from build123d import *

# Parameters (mm, degrees)
SKETCH_1_R          = 25
SKETCH_1_W          = 115
SKETCH_1_H          = 30
EXTRUDE_1_DEPTH     = 10
FILLET_1_R          = 20
SKETCH_2_R          = 18.75
CUT_EXTRUDE_1_DEPTH = 81.195074662
CUT_EXTRUDE_3_DEPTH = 81.195074662
FILLET_3_R          = 3
SKETCH_5_R          = 1.65
CUT_EXTRUDE_4_DEPTH = 81.195074662
SKETCH_6_R          = 1.65
CUT_EXTRUDE_5_DEPTH = 81.195074662
FILLET_5_R          = 5
SKETCH_7_R          = 18.75
SKETCH_7_R_2        = 16.75
EXTRUDE_2_DEPTH     = 2.3
CUT_EXTRUDE_6_DEPTH = 10
FILLET_6_R          = 3
SKETCH_9_R          = 1.65
CUT_EXTRUDE_7_DEPTH = 10


with BuildPart() as part:
    # ｽｹｯﾁ1 → ﾎﾞｽ - 押し出し1 (new body)
    with BuildSketch(Plane.XY):
        with Locations((30, 30)):
            Circle(SKETCH_1_R)
        with Locations((-30, 30)):
            Circle(SKETCH_1_R)
        Rectangle(SKETCH_1_W, SKETCH_1_H)
        with BuildLine():
            ThreePointArc((-50, 15), (-30, 5), (-10, 15))
            Line((-10, 15), (-50, 15))
        make_face()
        with BuildLine():
            Line((-50, 15), (-10, 15))
            ThreePointArc((-10, 15), (-6.282917549, 22.09430585), (-5, 30))
            ThreePointArc((-5, 30), (-12.32233047, 47.67766953), (-30, 55))
            ThreePointArc((-30, 55), (-47.67766953, 47.67766953), (-55, 30))
            ThreePointArc((-55, 30), (-53.717082451, 22.09430585), (-50, 15))
        make_face()
        with BuildLine():
            Line((-10, 15), (10, 15))
            ThreePointArc((10, 15), (7.639320225, 41.180339887), (30, 55))
            Line((30, 55), (-30, 55))
            ThreePointArc((-30, 55), (-12.32233047, 47.67766953), (-5, 30))
            ThreePointArc((-5, 30), (-6.282917549, 22.09430585), (-10, 15))
        make_face()
        with BuildLine():
            ThreePointArc((10, 15), (30, 5), (50, 15))
            Line((50, 15), (10, 15))
        make_face()
        with BuildLine():
            Line((10, 15), (50, 15))
            ThreePointArc((50, 15), (53.717082451, 22.09430585), (55, 30))
            ThreePointArc((55, 30), (47.67766953, 47.67766953), (30, 55))
            ThreePointArc((30, 55), (7.639320225, 41.180339887), (10, 15))
        make_face()
        with BuildLine():
            Line((50, 15), (57.5, 15))
            Line((57.5, 15), (55, 30))
            ThreePointArc((55, 30), (53.717082451, 22.09430585), (50, 15))
        make_face()
        with BuildLine():
            Line((-55, 30), (-57.5, 15))
            Line((-57.5, 15), (-50, 15))
            ThreePointArc((-50, 15), (-53.717082451, 22.09430585), (-55, 30))
        make_face()
    extrude(amount=EXTRUDE_1_DEPTH)

    # ﾌｨﾚｯﾄ1
    fillet_1_edges = [part.edges().sort_by_distance(p)[0] for p in [
        (55, 30, 5),
        (57.5, 15, 5),
        (-57.5, 15, 5),
        (-55, 30, 5),
    ]]
    fillet(fillet_1_edges, radius=FILLET_1_R)

    # ｽｹｯﾁ2 → ｶｯﾄ - 押し出し1 (cut, through all)
    with BuildSketch(Plane.XY.offset(10)):
        with Locations((30, 30)):
            Circle(SKETCH_2_R)
        with Locations(Location((-30, 30, 0), (0, 0, 180))):
            Circle(SKETCH_2_R)
    extrude(amount=-CUT_EXTRUDE_1_DEPTH, mode=Mode.SUBTRACT)

    # ｽｹｯﾁ4 → ｶｯﾄ - 押し出し3 (cut, through all)
    with BuildSketch(Plane(origin=(0, 0, 0), x_dir=(-1, 0, 0), z_dir=(0, 0, -1))):
        with BuildLine():
            Line((-5, -5), (-5, 15))
            Line((-5, 15), (-10, 15))
            ThreePointArc((-10, 15), (-28.103103333, 5.072068216), (-47.5, 12.146428929))
            Line((-47.5, 12.146428929), (-47.5, -5))
            Line((-47.5, -5), (-5, -5))
        make_face()
        with BuildLine():
            Line((10, 15), (5, 15))
            Line((5, 15), (5, -5))
            Line((5, -5), (47.5, -5))
            Line((47.5, -5), (47.5, 12.146428929))
            ThreePointArc((47.5, 12.146428929), (28.103103333, 5.072068216), (10, 15))
        make_face()
    extrude(amount=-CUT_EXTRUDE_3_DEPTH, mode=Mode.SUBTRACT)

    # ﾌｨﾚｯﾄ3
    fillet_3_edges = [part.edges().sort_by_distance(p)[0] for p in [
        (-47.5, 12.146428929, 5),
        (-47.5, -5, 5),
        (-5, -5, 5),
        (-5, 15, 5),
        (-10, 15, 5),
        (47.5, 12.146428929, 5),
        (10, 15, 5),
        (5, 15, 5),
        (5, -5, 5),
        (47.5, -5, 5),
    ]]
    fillet(fillet_3_edges, radius=FILLET_3_R)

    # ｽｹｯﾁ5 → ｶｯﾄ - 押し出し4 (cut, through all)
    with BuildSketch(Plane(origin=(0, 0, 0), x_dir=(-1, 0, 0), z_dir=(0, 0, -1))):
        with Locations((-30, 51.75)):
            Circle(SKETCH_5_R)
        with Locations((-14.620427509, 45.379572491)):
            Circle(SKETCH_5_R)
        with Locations((-8.25, 30)):
            Circle(SKETCH_5_R)
        with Locations((-14.620427509, 14.620427509)):
            Circle(SKETCH_5_R)
        with Locations((-30, 8.25)):
            Circle(SKETCH_5_R)
        with Locations((-45.379572491, 14.620427509)):
            Circle(SKETCH_5_R)
        with Locations((-51.75, 30)):
            Circle(SKETCH_5_R)
        with Locations((-45.379572491, 45.379572491)):
            Circle(SKETCH_5_R)
        with Locations(Location((45.379572491, 45.379572491, 0), (0, 0, 180))):
            Circle(SKETCH_5_R)
        with Locations(Location((51.75, 30, 0), (0, 0, 180))):
            Circle(SKETCH_5_R)
        with Locations(Location((45.379572491, 14.620427509, 0), (0, 0, 180))):
            Circle(SKETCH_5_R)
        with Locations(Location((30, 8.25, 0), (0, 0, 180))):
            Circle(SKETCH_5_R)
        with Locations(Location((14.620427509, 14.620427509, 0), (0, 0, 180))):
            Circle(SKETCH_5_R)
        with Locations(Location((8.25, 30, 0), (0, 0, 180))):
            Circle(SKETCH_5_R)
        with Locations(Location((14.620427509, 45.379572491, 0), (0, 0, 180))):
            Circle(SKETCH_5_R)
        with Locations(Location((30, 51.75, 0), (0, 0, 180))):
            Circle(SKETCH_5_R)
    extrude(amount=-CUT_EXTRUDE_4_DEPTH, mode=Mode.SUBTRACT)

    # ｽｹｯﾁ6 → ｶｯﾄ - 押し出し5 (cut, through all)
    with BuildSketch(Plane(origin=(0, 0, 0), x_dir=(-1, 0, 0), z_dir=(0, 0, -1))):
        with Locations((-52.5, -10)):
            Circle(SKETCH_6_R)
        with Locations(Location((52.5, -10, 0), (0, 0, 180))):
            Circle(SKETCH_6_R)
        with Locations((0, -5)):
            Circle(SKETCH_6_R)
    extrude(amount=-CUT_EXTRUDE_5_DEPTH, mode=Mode.SUBTRACT)

    # ﾌｨﾚｯﾄ5
    fillet_5_edges = [part.edges().sort_by_distance(p)[0] for p in [
        (57.5, -15, 5),
        (-57.5, -15, 5),
    ]]
    fillet(fillet_5_edges, radius=FILLET_5_R)

    # ｽｹｯﾁ7 → ﾎﾞｽ - 押し出し2 (add)
    # profile 1 of 2: a face of its own
    with BuildSketch(Plane.XY.offset(10)):
        with Locations((-30, 30)):
            Circle(SKETCH_7_R)
        with Locations((-30, 30)):
            Circle(SKETCH_7_R_2, mode=Mode.SUBTRACT)
    # profile 2 of 2: a face of its own
    with BuildSketch(Plane.XY.offset(10)):
        with Locations((30, 30)):
            Circle(SKETCH_7_R)
        with Locations((30, 30)):
            Circle(SKETCH_7_R_2, mode=Mode.SUBTRACT)
    extrude(amount=-EXTRUDE_2_DEPTH)

    # ｽｹｯﾁ8 → ｶｯﾄ - 押し出し6 (cut)
    with BuildSketch(Plane(origin=(0, 0, 0), x_dir=(-1, 0, 0), z_dir=(0, 0, -1))):
        with BuildLine():
            Line((-5.459217616, 20), (0, 20))
            Line((0, 20), (0, 50))
            Line((0, 50), (-12.614661349, 50))
            ThreePointArc((-12.614661349, 50), (-5.886088307, 40.989506944), (-3.5, 30))
            ThreePointArc((-3.5, 30), (-3.994416627, 24.904940293), (-5.459217616, 20))
        make_face()
        with BuildLine():
            Line((0, 50), (0, 20))
            Line((0, 20), (5.459217616, 20))
            ThreePointArc((5.459217616, 20), (4.223074151, 36.148178084), (12.614661349, 50))
            Line((12.614661349, 50), (0, 50))
        make_face()
    extrude(amount=-CUT_EXTRUDE_6_DEPTH, mode=Mode.SUBTRACT)

    # ﾌｨﾚｯﾄ6
    fillet_6_edges = [part.edges().sort_by_distance(p)[0] for p in [
        (-5.459217616, 20, 5),
        (5.459217616, 20, 5),
        (12.614661349, 50, 5),
        (-12.614661349, 50, 5),
    ]]
    fillet(fillet_6_edges, radius=FILLET_6_R)

    # ｽｹｯﾁ9 → ｶｯﾄ - 押し出し7 (cut)
    with BuildSketch(Plane.XZ.offset(15)):
        with Locations((-42.5, 5)):
            Circle(SKETCH_9_R)
        with Locations(Location((42.5, 5, 0), (0, 0, 180))):
            Circle(SKETCH_9_R)
    extrude(amount=-CUT_EXTRUDE_7_DEPTH, mode=Mode.SUBTRACT)


solid = part.part
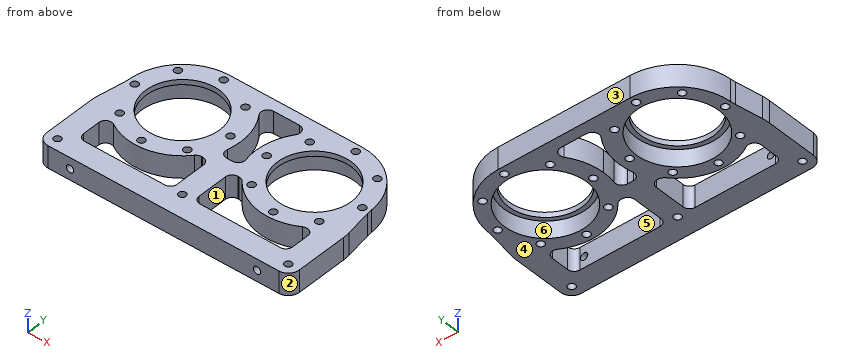
Build history of the part. All positions in model axes, mm. Face numbers are marked on the shaded views. A direction names the side the tool comes from. Round coordinates to 2 decimals unless told otherwise and drop trailing zeros. Loops run counter-clockwise (first coordinate to the right, second up) from the corner with the lowest first, then second, coordinate; pieces in that order, holes last. Notation, with made-up numbers: (56, 4.5) -> (111, 4.5) arc R16 ccw to (111, 10.5) -> close; hole circle Ø11 at (3.25, 35). An arc over 180 degrees is marked (long way). One line per item, written item: value. Start each with the question number.
Q1. Cut at C-C on y = 37.5. List the corners of the cut face in (x, z), plus the area to 3 significant figures.
Q2. Cut at D-D on z = 5. Count the separate pieces of the cut face and the enclosed holes in it, plus the area to 3 significant figures.
Q3. Cut at B-B on y = 1. List the corners of the cut face in (x, z).
Q4. Probe line 1 along X through (y, z) = (2, 4); line 2 along Y through (x, z) = (30, 5.25); line 3 along Y through (x, z) = (-30, 9.5). List the from-to ranges inside material, lowest first.
Q5. Two-plate mould, pull along Y, no slides. Class the marked faces 1, 2 and 3: released by +Y, released by -Y, zero draft, split by the parting line, or undercut.
Q6. Drop flat-ended pins along their axis: pin 1 Ø3 at (x, y) = (-30, 51.75) entering from -Z; pin 2 Ø2 at (x, z) = (42.5, 5) entering from +Y; pin 3 Ø1 at (y, z) = (29.5, 6) entering from +X. Give the stop position or say it passes through.
Q7. Cut at A-A on x = 0. List the corners of the cut face in (y, z), plus the area to 3 significant figures.
Q8. 3-axis set-ups, long thin cutter, end or side, ignore diameter. For the marked faces 4, 5 and 6: which of +Z, -Z, +X, -X, +Y, -Y reach the whole face in a straight line?
Computed:
1. outline: (-53.85, 0) -> (-47.18, 0) -> (-47.18, 7.7) -> (-44.98, 7.7) -> (-44.98, 10) -> (-53.85, 10) -> close; (-15.02, 7.7) -> (-12.82, 7.7) -> (-12.82, 0) -> (-4.58, 0) -> (-4.58, 10) -> (-15.02, 10) -> close; (4.58, 0) -> (12.82, 0) -> (12.82, 7.7) -> (15.02, 7.7) -> (15.02, 10) -> (4.58, 10) -> close; (44.98, 7.7) -> (47.18, 7.7) -> (47.18, 0) -> (53.85, 0) -> (53.85, 10) -> (44.98, 10) -> close
1. area: 318 mm²
2. separate pieces: 1
2. enclosed holes: 22
2. area: 3,740 mm²
3. outline: (-57.5, 0) -> (-47.5, 0) -> (-47.5, 10) -> (-57.5, 10) -> close; (-5, 0) -> (5, 0) -> (5, 10) -> (-5, 10) -> close; (47.5, 0) -> (57.5, 0) -> (57.5, 10) -> (47.5, 10) -> close
4. line 1: -57.5 to -47.5, -5 to 5, 47.5 to 57.5
4. line 2: -15 to -5, 5 to 6.6, 9.9 to 11.25, 48.75 to 50.1, 53.4 to 55
4. line 3: -15 to -5, 5 to 6.6, 9.9 to 13.25, 46.75 to 50.1, 53.4 to 55
5. face 1: undercut
5. face 2: released by -Y
5. face 3: released by +Y
6. pin 1: through
6. pin 2: y = 52.2
6. pin 3: x = 55.17
7. outline: (-15, 0) -> (-6.65, 0) -> (-6.65, 10) -> (-15, 10) -> close; (-3.35, 0) -> (20, 0) -> (20, 10) -> (-3.35, 10) -> close; (50, 0) -> (55, 0) -> (55, 10) -> (50, 10) -> close
7. area: 367 mm²
8. face 4: -Z, +X, -X, +Y, -Y
8. face 5: +Z, -Z
8. face 6: -Z
